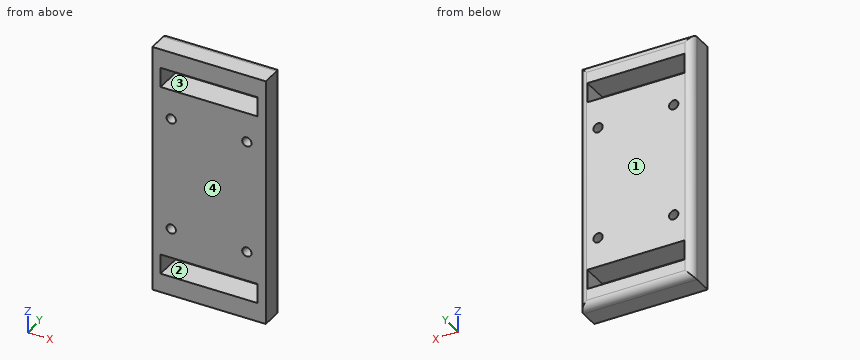
Autodesk Inventor part; units mm, degrees
ref_plane "YZ Plane" through (0, 0, 0) normal (1, 0, 0) x (0, 1, 0)
ref_plane "XZ Plane" through (0, 0, 0) normal (0, 1, 0) x (-1, 0, 0)
ref_plane "XY Plane" through (0, 0, 0) normal (0, 0, 1) x (1, 0, 0)
sketch "Sketch1" plane through (0, 0, 0) normal (0, 1, 0) x (-1, 0, 0)
  line L0 (0, 0) -> (30, 0)
  line L1 (30, 0) -> (30, -65.85)
  line L2 (30, -65.85) -> (0, -65.85)
  line L3 (0, -65.85) -> (0, 0)
  dimension "d0" = 30
  dimension "d1" = 65.85
extrude "Extrusion1" add sketch "Sketch1" along normal blind 7
sketch "Sketch2" plane through (0, 7, 0) normal (0, 1, 0) x (1, 0, 0)
  line L0 (-27.82, 5) -> (-2.18, 5)
  line L1 (-2.18, 5) -> (-2.18, 10.2)
  line L2 (-2.18, 10.2) -> (-27.82, 10.2)
  line L3 (-27.82, 10.2) -> (-27.82, 5)
  line L4 (-27.82, 55.65) -> (-2.18, 55.65)
  line L5 (-2.18, 55.65) -> (-2.18, 60.85)
  line L6 (-2.18, 60.85) -> (-27.82, 60.85)
  line L7 (-27.82, 60.85) -> (-27.82, 55.65)
  line L8 (-30, 0) -> (0, 0)
  line L9 (-15, 10.2) -> (-15, 55.65) construction
  line L10 (-30, 65.85) -> (-30, 0) construction
  line L11 (0, 65.85) -> (-30, 65.85) construction
  point P0 (-15, 5)
  point P1 (-15, 0)
  point P2 (-15, 32.925)
  point P3 (-30, 32.925)
  dimension "d4" = 25.64
  dimension "d5" = 5.2
  dimension "d6" = 5
extrude "Extrusion2" cut sketch "Sketch2" against normal up to next
sketch "Sketch3" plane through (0, 0, 0) normal (0, -1, 0) x (1, 0, 0)
  line L0 (-25, -47.85) -> (-5, -18) construction
  line L1 (-30, -65.85) -> (0, -65.85) construction
  line L2 (0, -65.85) -> (0, 0) construction
  point P0 (-25, -18)
  point P1 (-5, -47.85)
  point P2 (-15, -32.925)
  point P3 (-15, -65.85)
  point P4 (0, -32.925)
  dimension "d9" = 29.85
  dimension "d10" = 20
hole "Hole1" at (-25, 0, -47.85) at (-25, 0, -18) at (-5, 0, -18) at (-5, 0, -47.85) direction (0, 1, 0) diameter 2.46 end through all
fillet "Fillet1" radius 2 4 edges at (-30, 7, -32.925) (0, 7, -32.925) (-15, 7, -65.85) (-15, 7, 0)
properties part number "Tilt_Camera_Mount_Plate"
The model under review builds one solid part; all positions refer to its coordinate system, in mm. Face numbers are marked on the shaded views. A direction names the side the tool comes from. Round coordinates to 2 decimals unless told otherwise and drop trailing zeros. Loops run counter-clockwise (first coordinate to the right, second up) from the corner with the lowest first, then second, coordinate; pieces in that order, holes last.
1) Wall thickness on line 1 along X through (y, z) = (3.5, -18); line 2 along Z through (x, y) = (-27.75, 4.75); line 3 along Z through (x, y) = (-25, 2.75): over which ranges is each line inside the solid? List them lowest first.
Values follow:
line 1: x = -30 to -26.23, -23.77 to -6.23, -3.77 to 0
line 2: z = -65.85 to -60.85, -55.65 to -10.2, -5 to 0
line 3: z = -65.85 to -60.85, -55.65 to -49.08, -46.62 to -19.23, -16.77 to -10.2, -5 to 0
2) The part is to be moulded in two halves that separate along Z. For the marked faces 1 and 2, say which applies: pulls with the +Z half, pulls with the -Z half, needs draft (parallel to the pull), parting line crosses it, or undercut.
Values follow:
face 1: needs draft
face 2: undercut
3) Consider section D-D on y = 3.5. State the section outline as (x, z) points, then the cut area to 3 significant figures.
Values follow:
outline: (-30, -65.85) - (0, -65.85) - (0, 0) - (-30, 0) - close; hole (-27.82, -60.85) - (-2.18, -60.85) - (-2.18, -55.65) - (-27.82, -55.65) - close; hole (-27.82, -10.2) - (-2.18, -10.2) - (-2.18, -5) - (-27.82, -5) - close; hole circle Ø2.46 at (-25, -47.85); hole circle Ø2.46 at (-25, -18); hole circle Ø2.46 at (-5, -47.85); hole circle Ø2.46 at (-5, -18)
area: 1,690 mm2
4) Consider section C-C on x = -14.25. State the section outline as (y, z) points.
Values follow:
outline: (0, -65.85) - (5, -65.85) arc R2 ccw to (7, -63.85) - (7, -60.85) - (0, -60.85) - close; (0, -55.65) - (7, -55.65) - (7, -10.2) - (0, -10.2) - close; (0, -5) - (7, -5) - (7, -2) arc R2 ccw to (5, 0) - (0, 0) - close
5) Tool access review of the marked faces 3 and 4: name each direction out of +Z, -Z, +X, -X, +Y, -Y from which nothing blocks a thin tool from reaching the whole face with its end or side.
Values follow:
face 3: +Y, -Y
face 4: +Z, -Z, +X, -X, -Y
6) Consider section A-A on x = -5. State the section outline as (y, z) points.
Values follow:
outline: (0, -65.85) - (5, -65.85) arc R2 ccw to (7, -63.85) - (7, -60.85) - (0, -60.85) - close; (0, -55.65) - (7, -55.65) - (7, -49.08) - (0, -49.08) - close; (0, -46.62) - (7, -46.62) - (7, -19.23) - (0, -19.23) - close; (0, -16.77) - (7, -16.77) - (7, -10.2) - (0, -10.2) - close; (0, -5) - (7, -5) - (7, -2) arc R2 ccw to (5, 0) - (0, 0) - close
7) Consider section B-B on z = -18. State the section outline as (x, y) points.
Values follow:
outline: (-30, 0) - (-26.23, 0) - (-26.23, 7) - (-28, 7) arc R2 ccw to (-30, 5) - close; (-23.77, 0) - (-6.23, 0) - (-6.23, 7) - (-23.77, 7) - close; (-3.77, 0) - (0, 0) - (0, 5) arc R2 ccw to (-2, 7) - (-3.77, 7) - close
8) Clearance check with a flat-ended pin moving along its axis: P1, Ø3.5, axis at x = -19.5, y = 4, coming from the +Z side. State where the tip first meets the part, or that it passes through.
Values follow:
P1: stops at z = 0
